```python
from build123d import *

# Parameters (mm, degrees)
SKETCH_1_R          = 1
EXTRUDE_1_DEPTH     = 2
SKETCH_2_W          = 1.3
SKETCH_2_H          = 56
EXTRUDE_2_DEPTH     = 3
SKETCH_3_W          = 10
SKETCH_3_H          = 11
SKETCH_3_W_2        = 20
SKETCH_3_H_2        = 14
CUT_EXTRUDE_1_DEPTH = 1.2
SKETCH_6_W          = 4.5
SKETCH_6_H          = 8
CUT_EXTRUDE_4_DEPTH = 1.2
SKETCH_4_W          = 1.3
SKETCH_4_H          = 3.5
CUT_EXTRUDE_2_DEPTH = 1
SKETCH_5_W          = 48
SKETCH_5_H          = 37
CUT_EXTRUDE_3_DEPTH = 2


with BuildPart() as part:
    # Sketch 1 → Extrude 1 (new body)
    with BuildSketch(Plane.XY):
        Polygon((18.5, 15), (-18.5, 15), (-18.5, 17), (-17, 18.5), (-17, 28), (-33, 28), (-33, -28), (-18.5, -28), (-18.5, -17), (-18.5, -15), (18.5, -15), (18.5, -17), (17, -18.5), (17, -28), (33, -28), (33, 28), (17, 28), (17, 18.5), (18.5, 17), align=None)
        with Locations((19, -20)):
            Circle(SKETCH_1_R, mode=Mode.SUBTRACT)
        with Locations((-19, 20)):
            Circle(SKETCH_1_R, mode=Mode.SUBTRACT)
        with Locations((19, 20)):
            Circle(SKETCH_1_R, mode=Mode.SUBTRACT)
    extrude(amount=EXTRUDE_1_DEPTH)

    # Sketch 2 → Extrude 2 (add)
    with BuildSketch(Plane.XY.offset(2)):
        with Locations((-32.35, 0)):
            Rectangle(SKETCH_2_W, SKETCH_2_H)
        with Locations((32.35, 0)):
            Rectangle(SKETCH_2_W, SKETCH_2_H)
        with Locations((-29.35, 0)):
            Rectangle(SKETCH_2_W, SKETCH_2_H)
        with Locations((-26.35, 0)):
            Rectangle(SKETCH_2_W, SKETCH_2_H)
        with Locations((-23.35, 0)):
            Rectangle(SKETCH_2_W, SKETCH_2_H)
        with Locations((29.35, 0)):
            Rectangle(SKETCH_2_W, SKETCH_2_H)
        with Locations((26.35, 0)):
            Rectangle(SKETCH_2_W, SKETCH_2_H)
        with Locations((23.35, 0)):
            Rectangle(SKETCH_2_W, SKETCH_2_H)
    extrude(amount=EXTRUDE_2_DEPTH)

    # Sketch 3 → Cut-Extrude 1 (cut)
    with BuildSketch(Plane(origin=(0, 0, 0), x_dir=(-1, 0, 0), z_dir=(0, 0, -1))):
        Polygon((-15, -3), (-15, 15), (-18.5, 15), (-33, 15), (-33, -3), (-23, -3), align=None)
        with Locations((-28, -8.5)):
            Rectangle(SKETCH_3_W, SKETCH_3_H)
        with Locations((0, 4)):
            Rectangle(SKETCH_3_W_2, SKETCH_3_H_2)
    extrude(amount=-CUT_EXTRUDE_1_DEPTH, mode=Mode.SUBTRACT)

    # Sketch 6 → Cut-Extrude 4 (cut)
    with BuildSketch(Plane(origin=(0, 0, 0), x_dir=(-1, 0, 0), z_dir=(0, 0, -1))):
        with Locations((27.25, -24)):
            Rectangle(SKETCH_6_W, SKETCH_6_H)
    extrude(amount=-CUT_EXTRUDE_4_DEPTH, mode=Mode.SUBTRACT)

    # Sketch 4 → Cut-Extrude 2 (cut)
    with BuildSketch(Plane.XY.offset(5)):
        with Locations((32.35, -10.25)):
            Rectangle(SKETCH_4_W, SKETCH_4_H)
    extrude(amount=-CUT_EXTRUDE_2_DEPTH, mode=Mode.SUBTRACT)

    # Sketch 5 → Cut-Extrude 3 (cut)
    with BuildSketch(Plane.XY.offset(5)):
        Rectangle(SKETCH_5_W, SKETCH_5_H)
    extrude(amount=-CUT_EXTRUDE_3_DEPTH, mode=Mode.SUBTRACT)


solid = part.part
```
Work out the finished part from the listing and answer in its coordinate system (mm). A direction names the side the tool comes from. Round coordinates to 2 decimals unless told otherwise and drop trailing zeros. Loops run counter-clockwise (first coordinate to the right, second up) from the corner with the lowest first, then second, coordinate; pieces in that order, holes last. Notation, with made-up numbers: M 61.25,-15 L 119.25,-15 A13 ccw 119.25,-4 Z; hole C -24.5,63.25 d8. An arc over 180 degrees is marked long. Use CSV: the item, a comma, the result in double quotes.
Q1. Each of these flat-tipped pins is pushed along its axis until it touches: pin 1 (1 mm diameter, centred on x = 2.5, z = 1, fed in from -Y); pin 2 (1 mm diameter, centred on x = -12, y = -1.5, fed in from -Z); pin 3 (0.5 mm diameter, centred on x = 28, y = 3, fed in from +Z); pin 4 (0.6 mm diameter, centred on x = -3, z = 0.5, fed in from +Y). Where does it stop, or does it pass through?
Determined:
pin 1,"y = -15"
pin 2,"z = 0"
pin 3,"z = 2"
pin 4,"y = 15"
Q2. Section B-B, the plane x = -12.5 is taken. Determine the outline of the cut face in (y, z).
Determined:
outline,"M -15,0 L 15,0 L 15,2 L -15,2 Z"
Q3. Section A-A, the plane x = 7 is taken. Determine the outline of the cut face in (y, z).
Determined:
outline,"M -15,0 L -3,0 L -3,1.2 L 11,1.2 L 11,0 L 15,0 L 15,2 L -15,2 Z"
Q4. Consider L1, parallel to Y at x = 19, z = 0.75; L2, parallel to X at y = -0.5, z = 3.5; L3, parallel to Y at x = 19, z = 1.55. Determine where each line is inside the solid, lowest interval first.
Determined:
L1,"-28 to -21, -19 to -3, 15 to 19, 21 to 28"
L2,"-33 to -31.7, -30 to -28.7, -27 to -25.7, 25.7 to 27, 28.7 to 30, 31.7 to 33"
L3,"-28 to -21, -19 to 19, 21 to 28"
Q5. The mould has two halves that part along X. Classify faces 1 (the flat face through (-8, -6, 0)), 2 (the flat face through (28.7, 0, 3)), 3 (the flat face through (-33, 0, 2)): pulls with the +X half, pulls with the -X half, needs draft (parallel to the pull), parting line crosses it, or undercut.
Determined:
face 1,"needs draft"
face 2,"undercut"
face 3,"pulls with the -X half"
Q6. A tool of negligible diameter and unlimited length cuts with its end or side. For faces 4 (the flat face through (17.8, -17.7, 1)), 5 (the flat face through (27, 0, 3)), 6 (the flat face through (-27, -24, 1.2)), 7 (the flat face through (-17, 23, 1)), 8 (the flat face through (0, 4, 1.2)), from which of +Z, -Z, +X, -X, +Y, -Y can it reach the whole face along a straight path? Write none if from no direction.
Determined:
face 4,"+Z, -Z"
face 5,"+Z, +Y, -Y"
face 6,"-Z, -Y"
face 7,"+Z, -Z, +Y"
face 8,"-Z"
